from build123d import *

# Parameters (mm, degrees)
BOSS_EXTRUDE2_DEPTH = 1.4
SKETCH3_W           = 11
SKETCH3_H           = 6.5
BOSS_EXTRUDE4_DEPTH = 5.48
SKETCH4_W           = 10.6
SKETCH4_H           = 5.08
CUT_EXTRUDE1_DEPTH  = 5.98
SKETCH6_W           = 1
SKETCH6_H           = 2
CUT_EXTRUDE2_DEPTH  = 11.98
SKETCH7_W           = 1
SKETCH7_H           = 0.9
CUT_EXTRUDE3_DEPTH  = 1
SKETCH8_R           = 5
BOSS_EXTRUDE5_DEPTH = 5.48
SKETCH9_R           = 0.5
CUT_EXTRUDE4_DEPTH  = 5.48
SKETCH10_R          = 1
BOSS_EXTRUDE6_DEPTH = 1


with BuildPart() as part:
    # Sketch1 → Boss-Extrude2 (new body)
    with BuildSketch(Plane.XY):
        with BuildLine():
            Line((3.31662479, -5), (-3.31662479, -5))
            ThreePointArc((-3.31662479, -5), (-5.286764074, -2.837274331), (-6, 0))
            Line((-6, 0), (-6, 14))
            Line((-6, 14), (6, 14))
            Line((6, 14), (6, 0))
            ThreePointArc((6, 0), (5.286764074, -2.837274331), (3.31662479, -5))
        make_face()
    extrude(amount=BOSS_EXTRUDE2_DEPTH)

    # Sketch3 → Boss-Extrude4 (add)
    with BuildSketch(Plane.XY.offset(1.4)):
        with Locations((0, 10.25)):
            Rectangle(SKETCH3_W, SKETCH3_H)
    extrude(amount=BOSS_EXTRUDE4_DEPTH)

    # Sketch4 → Cut-Extrude1 (cut)
    with BuildSketch(Plane(origin=(0, 13.5, 0), x_dir=(1, 0, 0), z_dir=(0, 1, 0))):
        with Locations((0, -4.14)):
            Rectangle(SKETCH4_W, SKETCH4_H)
    extrude(amount=-CUT_EXTRUDE1_DEPTH, mode=Mode.SUBTRACT)

    # Sketch6 → Cut-Extrude2 (cut)
    with BuildSketch(Plane(origin=(5.5, 0, 0), x_dir=(0, 0, -1), z_dir=(1, 0, 0))):
        with Locations((-4.24, 12.5)):
            Rectangle(SKETCH6_W, SKETCH6_H)
    extrude(amount=-CUT_EXTRUDE2_DEPTH, mode=Mode.SUBTRACT)

    # Sketch7 → Cut-Extrude3 (cut)
    with BuildSketch(Plane.XY.offset(6.88)):
        with Locations((2.5, 7.45)):
            Rectangle(SKETCH7_W, SKETCH7_H)
        with Locations((1, 7.45)):
            Rectangle(SKETCH7_W, SKETCH7_H)
        with Locations((-1, 7.45)):
            Rectangle(SKETCH7_W, SKETCH7_H)
        with Locations((-2.5, 7.45)):
            Rectangle(SKETCH7_W, SKETCH7_H)
        with Locations((-4, 7.45)):
            Rectangle(SKETCH7_W, SKETCH7_H)
        with Locations((4, 7.45)):
            Rectangle(SKETCH7_W, SKETCH7_H)
    extrude(amount=-CUT_EXTRUDE3_DEPTH, mode=Mode.SUBTRACT)

    # Sketch8 → Boss-Extrude5 (add)
    with BuildSketch(Plane.XY.offset(1.4)):
        with Locations(Location((0, 0, 0), (0, 0, 270))):
            Circle(SKETCH8_R)
    extrude(amount=BOSS_EXTRUDE5_DEPTH)

    # Sketch9 → Cut-Extrude4 (cut)
    with BuildSketch(Plane.XY.offset(6.88)):
        Circle(SKETCH9_R)
    extrude(amount=-CUT_EXTRUDE4_DEPTH, mode=Mode.SUBTRACT)

    # Sketch10 → Boss-Extrude6 (add)
    with BuildSketch(Plane(origin=(0, 0, 0), x_dir=(-1, 0, 0), z_dir=(0, 0, -1))):
        Circle(SKETCH10_R)
    extrude(amount=BOSS_EXTRUDE6_DEPTH)


solid = part.part
Geometry: final body of the model. Coordinates: model frame, mm. A direction names the side the tool comes from. Give positions to 0.01 mm unless a question says otherwise; leave off trailing zeros. Write each loop counter-clockwise with the first axis right and the second up, starting at its lowest first coordinate (ties: lowest second). Pieces come first, ordered by that corner, then holes. Notation, with made-up numbers: (63.25, 68.5) - (71.25, 68.5) arc R33 cw to (71.25, 103.5) - close; hole circle Ø4 at (-14, 24.25). An arc over 180 degrees is marked (long way). Return JSON: item names as keys, results as strings. Group by question number.
1) Section C-C on z = 2.25. Return the cut outline in (x, y).
2) Mould query, pull axis Y, two halves, no side actions, for faces 6 (the flat face through (0, 0, 1.4)), 7 (the flat face through (0, -1, 6.88)), 8 (the flat face through (0, 14, 1)). Classes: released by +Y, released by -Y, zero draft, split by the parting line, or undercut.
3) First-contact query: P1, Ø1, axis at x = -3, y = 1, coming from the -Z side; P2, Ø0.6, axis at x = -4, y = 7.5, coming from the +Z side; P3, Ø1, axis at y = 7, z = 6.5, coming from the -X side; P4, Ø6, axis at x = -1, y = -0.5, coming from the -Z side. Flat tips, straight axial feed; report the tip coordinate or a pass-through.
4) Section A-A on z = 6.25. State how many separate pieces and enclosed holes the cut face has, plus the area to 3 significant figures.
5) Section B-B on y = 12.75. Return the cut outline in (x, z).
6) Line query: line 1 (Z direction, x = 3, y = 11.75); line 2 (X direction, y = 13, z = 6); line 3 (Z direction, x = 0, y = 7.25). Output: solid intervals per line, ascending.
7) Set-up query: faces 1 (the flat face through (-5.5, 10, 4)), 2 (the flat face through (5.5, 10, 4)), 3 (the flat face through (0, 7.52, 4)), 4 (the flat face through (0, 10, 6.88)), 5 (the flat face through (0.5, 7.3, 6.5)). Return all of +Z, -Z, +X, -X, +Y, -Y with unobstructed straight access to the full face (end or side cutting, diameter ignored); none if empty.
8) Section D-D on x = 4. Return the cut outline in (y, z), plus the area to 3 significant figures.
Filled in:
{
 "1": {"outline": "(-5.5, 7) - (5.5, 7) - (5.5, 13.5) - (5.3, 13.5) - (5.3, 7.52) - (-5.3, 7.52) - (-5.3, 13.5) - (-5.5, 13.5) - close; circle Ø10 at (0, 0); hole circle Ø1 at (0, 0)"},
 "2": {"face 6": "undercut", "face 7": "zero draft", "face 8": "released by +Y"},
 "3": {"P1": "stops at z = 0", "P2": "stops at z = 5.88", "P3": "stops at x = -5.5", "P4": "stops at z = -1"},
 "4": {"separate pieces": "8", "enclosed holes": "1", "area": "82.7 mm^2"},
 "5": {"outline": "(-6, 0) - (6, 0) - (6, 1.4) - (5.5, 1.4) - (5.5, 3.74) - (5.3, 3.74) - (5.3, 1.6) - (-5.3, 1.6) - (-5.3, 3.74) - (-5.5, 3.74) - (-5.5, 1.4) - (-6, 1.4) - close; (-5.5, 4.74) - (-5.3, 4.74) - (-5.3, 6.68) - (5.3, 6.68) - (5.3, 4.74) - (5.5, 4.74) - (5.5, 6.88) - (-5.5, 6.88) - close"},
 "6": {"line 1": "z = 0 to 1.6, 6.68 to 6.88", "line 2": "x = -5.5 to -5.3, 5.3 to 5.5", "line 3": "z = 0 to 6.88"},
 "7": {"face 1": "+Z, -X, +Y, -Y", "face 2": "+Z, +X, +Y, -Y", "face 3": "+Y", "face 4": "+Z, +X, -X, +Y, -Y", "face 5": "+Z"},
 "8": {"outline": "(-4.47, 0) - (14, 0) - (14, 1.4) - (13.5, 1.4) - (13.5, 1.6) - (7.52, 1.6) - (7.52, 5.88) - (7, 5.88) - (7, 1.4) - (3, 1.4) - (3, 6.88) - (-3, 6.88) - (-3, 1.4) - (-4.47, 1.4) - close; (7.9, 6.68) - (13.5, 6.68) - (13.5, 6.88) - (7.9, 6.88) - close", "area": "63.4 mm^2"}
}
